For this review, take the finished solid that the model builds, in its own axes (mm). Give positions to 0.01 mm unless a question says otherwise; leave off trailing zeros. Order: outer loops, then holes, each group sorted by start corner. A loop starts at its lowest first (then second) coordinate and runs counter-clockwise, first axis right, second up. Notation, with made-up numbers: (71, 76) - (117, 76) arc R35 ccw to (117, 115) - close; hole circle Ø8 at (33, 69.25). An arc over 180 degrees is marked (long way). One line per item, written item: value.
Autodesk Inventor part; units mm, degrees
ref_plane "YZ Plane" through (0, 0, 0) normal (1, 0, 0) x (0, 1, 0)
ref_plane "XZ Plane" through (0, 0, 0) normal (0, 1, 0) x (-1, 0, 0)
ref_plane "XY Plane" through (0, 0, 0) normal (0, 0, 1) x (1, 0, 0)
sketch "Sketch1" plane through (0, 0, 0) normal (0, 1, 0) x (-1, 0, 0)
  line L0 (0, -5) -> (0, -5)
  line L1 (5, 0) -> (5, 0)
  line L2 (0, 5) -> (0, 5)
  line L3 (-5, 0) -> (-5, 0)
  line L4 (-5, -5) -> (5, 5) construction
  line L5 (5, -5) -> (-5, 5) construction
  circle A0 centre (0, 0) radius 2.5
  arc A1 (0, 5) -> (-5, 0) centre (0, 0) ccw
  arc A2 (5, 0) -> (0, 5) centre (0, 0) ccw
  arc A3 (0, -5) -> (5, 0) centre (0, 0) ccw
  arc A4 (-5, 0) -> (0, -5) centre (0, 0) ccw
  point P0 (0, 5)
  point P1 (-5, 0)
  dimension "d0" = 10
  dimension "d1" = 10
  dimension "d46" = 5
  dimension "d47" = 5
extrude "Extrusion1" add sketch "Sketch1" along normal blind 5
equation "\"BendRadius\" = Thickness"
equation "\"BendReliefWidth\" = Thickness"
equation "\"BendReliefDepth\" = 0.5 * Thickness"
equation "\"CornerReliefSize\" = 4 * Thickness"
equation "\"MinimumRemnant\" = 2 * Thickness"
equation "\"TransitionRadius\" = BendRadius"
equation "\"JacobiRadiusSize\" = BendRadius"
equation "\"GapSize\" = Thickness"
properties part number "base"
(1) For P1, Ø1.5, axis at x = 1.5, y = 1, coming from the +Z side, flat-tipped, find the tip position at first contact; note if it passes through.
Answers below:
P1: stops at z = 4.94
(2) Take a section at C-C (y = 0.9). Write out the cut boundary in (x, z).
Answers below:
outline: circle Ø10 at (0, 0); hole circle Ø5 at (0, 0)
(3) Take a section at D-D (x = -3). Write out the cut boundary in (y, z), then the cut area to 3 significant figures.
Answers below:
outline: (0, -4) - (5, -4) - (5, 4) - (0, 4) - close
area: 40.0 mm^2
(4) Take a section at A-A (x = 0). Write out the cut boundary in (y, z).
Answers below:
outline: (0, -5) - (5, -5) - (5, -2.5) - (0, -2.5) - close; (0, 2.5) - (5, 2.5) - (5, 5) - (0, 5) - close
(5) Wall thickness on line 1 (Z direction, x = 0, y = 2.15); line 2 (Z direction, x = 2.25, y = 4); line 3 (X direction, y = 2.9, z = -1): over which ranges is each line inside the solid? List them lowest first. Write a range as from..to.
Answers below:
line 1: z = -5..-2.5, 2.5..5
line 2: z = -4.47..-1.09, 1.09..4.47
line 3: x = -4.9..-2.29, 2.29..4.9
(6) Draft analysis for pull direction X (two halves, no side actions). For faces 1 (the face through (0.54, 2.46, 2.44)), 2 (the face through (-2, 5, -2)), 3 (the face through (-1.08, 2.46, -4.88)), state which applies: pulls with the +X half, pulls with the -X half, needs draft (parallel to the pull), parting line crosses it, or undercut.
Answers below:
face 1: undercut
face 2: needs draft
face 3: parting line crosses it
(7) Take a section at B-B (z = 0). Write out the cut boundary in (x, y), then the cut area to 3 significant figures.
Answers below:
outline: (-5, 0) - (-2.5, 0) - (-2.5, 5) - (-5, 5) - close; (2.5, 0) - (5, 0) - (5, 5) - (2.5, 5) - close
area: 25.0 mm^2
